Geometry: see drawing. Coordinates: mm, zero at the bounding-box minimum. Coordinates: 2 decimals unless noted, no trailing zeros. Write each loop counter-clockwise with the first axis right and the second up, starting at its lowest first coordinate (ties: lowest second). Pieces come first, ordered by that corner, then holes. Notation, with made-up numbers: (43.25, -25) -> (61.25, -25) arc R15 cw to (61.25, -11) -> close; hole circle Ø8 at (68, -26.5). An arc over 180 degrees is marked (long way). Answer as a JSON object with one key per item and string values. Group by question number.
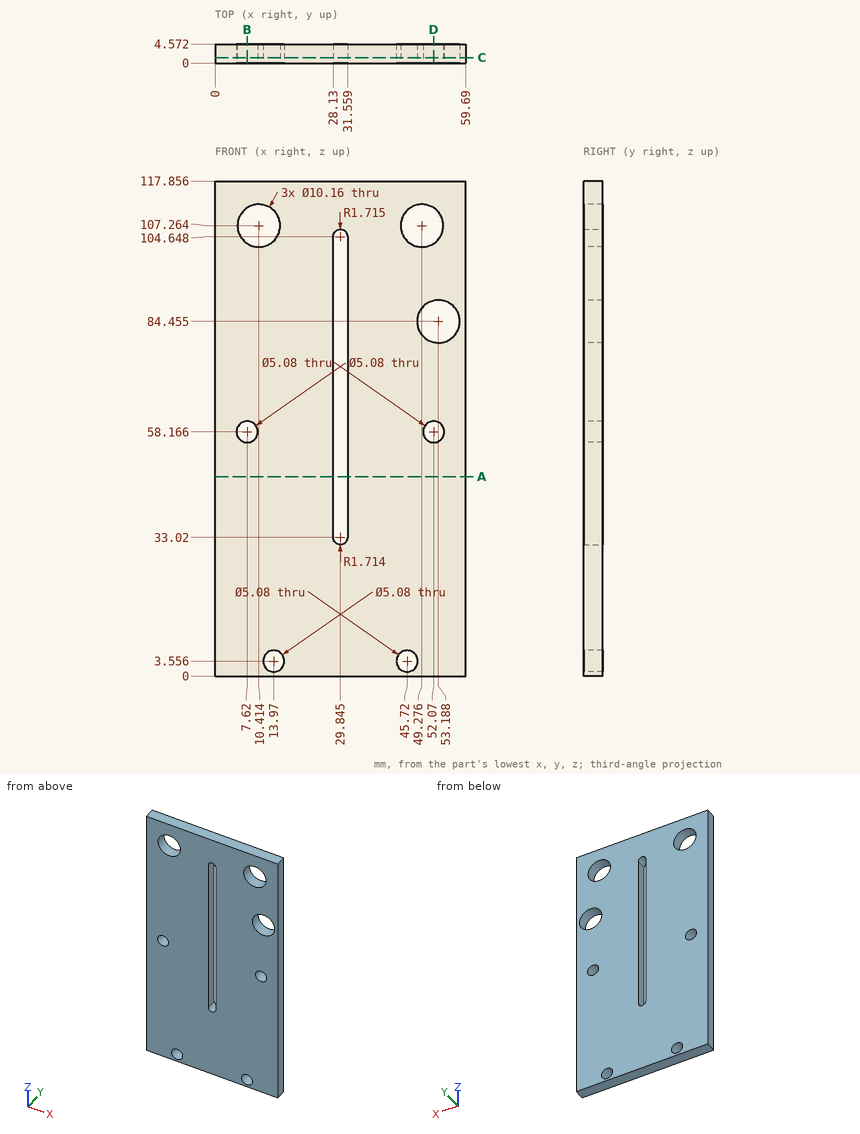
Item 1: Contact query for a flat-ended pin moving along its axis: pin 1 (6 mm diameter, centred on x = 53.19, z = 84.46, fed in from +Y). Output: stop coordinate, or through.
Item 2: Section D-D on x = 52.07. Output: boundary loops of the cut face in (y, z) (1 decimal).
Item 3: Ray query, L1, parallel to X at y = 1.45, z = 45; L2, parallel to Z at x = 45.72, y = 2.35 (1 decimal); L3, parallel to Z at x = 13, y = 3.2 (1 decimal). Return the intervals inside material, ascending. Write a range as [from, to].
Item 4: Section A-A on z = 47.5. Output: boundary loops of the cut face in (x, y).
Item 5: Section C-C on y = 1.3. Give the number of separate pieces and of enclosed holes in the cut face.
Item 6: Section B-B on x = 7.62. Output: boundary loops of the cut face in (y, z) (1 decimal), then the cut area to 3 significant figures.
Answer sheet:
{
 "1": {"pin 1": "passes through"},
 "2": {"outline": "(0, 0) -> (4.6, 0) -> (4.6, 55.6) -> (0, 55.6) -> close; (0, 60.7) -> (4.6, 60.7) -> (4.6, 79.5) -> (0, 79.5) -> close; (0, 89.4) -> (4.6, 89.4) -> (4.6, 103) -> (0, 103) -> close; (0, 111.5) -> (4.6, 111.5) -> (4.6, 117.9) -> (0, 117.9) -> close"},
 "3": {"L1": "x = [0, 28.13], [31.56, 59.69]", "L2": "z = [0, 1], [6.1, 103.6], [110.9, 117.9]", "L3": "z = [0, 1.2], [5.9, 102.9], [111.6, 117.9]"},
 "4": {"outline": "(0, 0) -> (28.13, 0) -> (28.13, 4.57) -> (0, 4.57) -> close; (31.56, 0) -> (59.69, 0) -> (59.69, 4.57) -> (31.56, 4.57) -> close"},
 "5": {"separate pieces": "1", "enclosed holes": "8"},
 "6": {"outline": "(0, 0) -> (4.6, 0) -> (4.6, 55.6) -> (0, 55.6) -> close; (0, 60.7) -> (4.6, 60.7) -> (4.6, 103) -> (0, 103) -> close; (0, 111.5) -> (4.6, 111.5) -> (4.6, 117.9) -> (0, 117.9) -> close", "area": "477 mm^2"}
}
